Input: part model. Units: mm. Frame: model coordinates. Coordinates: 2 decimals unless noted, no trailing zeros. Loops run counter-clockwise (first coordinate to the right, second up) from the corner with the lowest first, then second, coordinate; pieces in that order, holes last. Notation, with made-up numbers: (5.25, 38) - (52.25, 38) arc R26 cw to (52.25, 58) - close; hole circle Ø6 at (33, 56.25). An arc over 180 degrees is marked (long way). Use a Markdown table: item, result. Add a question column.
1. Draft query along Y for faces 1 (the face through (-1, 1, 0)), 2 (the face through (0.221, -18.314, 0.606)), 3 (the face through (-8.67, -39.05, 1.48)). Return one class per face: released by +Y, released by -Y, zero draft, split by the parting line, or undercut.
2. Section query C-C on y = -20. Return the cut outline in (x, z), then the cut area to 3 significant figures.
3. Contact query for flat-ended pins moving along their axis: P1, Ø4.5, axis at x = 20, y = 0, coming from the +Z side; P2, Ø4, axis at x = 0, y = -20, coming from the +Z side; P3, Ø2.5, axis at x = 0, y = 20, coming from the +Z side; P4, Ø1, axis at y = -26.5, z = 1, coming from the +X side. Output: stop coordinate, or through.
4. Section query A-A on z = 1.8. Return the cut outline in (x, y).
5. Section query B-B on x = 0. Return the cut outline in (y, z).
6. Ray query, L1, parallel to Y at x = 0, z = 0.7; L2, parallel to Y at x = -20, z = 0.75. Return the intervals inside material, ascending. Write a range as [from, to].
```python
from build123d import *

# Parameters (mm, degrees)
SKETCH_1_R                   = 40
EXTRUDE_1_DEPTH              = 3
HOLE_WIZARD_M3_1_D           = 3.4
HOLE_WIZARD_M3_1_DEPTH       = 10.12
HOLE_WIZARD_M3_1_CSINK_D     = 6.94
HOLE_WIZARD_M3_1_CSINK_ANGLE = 90
HOLE_WIZARD_M3_1_TIP         = 1.021463052


with BuildPart() as part:
    # 草图1 → 凸台-拉伸1 (new body)
    with BuildSketch(Plane.XY):
        Circle(SKETCH_1_R)
    extrude(amount=EXTRUDE_1_DEPTH)

    # M3 六角凹锥坑头螺钉的锥形沉头孔1
    with Locations(Plane(origin=(0, 20, 3), x_dir=(1, 0, 0), z_dir=(0, 0, 1))):
        with Locations((0, 0), (20, -20), (0, -40), (-20, -20)):
            CounterSinkHole(HOLE_WIZARD_M3_1_D / 2, HOLE_WIZARD_M3_1_CSINK_D / 2, depth=HOLE_WIZARD_M3_1_DEPTH, counter_sink_angle=HOLE_WIZARD_M3_1_CSINK_ANGLE)
            with Locations((0, 0, -(HOLE_WIZARD_M3_1_DEPTH + HOLE_WIZARD_M3_1_TIP / 2))):  # 118° drill point
                Cone(0, HOLE_WIZARD_M3_1_D / 2, HOLE_WIZARD_M3_1_TIP, mode=Mode.SUBTRACT)


solid = part.part
```
Resolved:
| question | item | result |
|---|---|---|
| 1 | face 1 | zero draft |
| 1 | face 2 | undercut |
| 1 | face 3 | split by the parting line |
| 2 | outline | (-34.64, 0) - (-1.7, 0) - (-1.7, 1.23) - (-3.47, 3) - (-34.64, 3) - close; (1.7, 0) - (34.64, 0) - (34.64, 3) - (3.47, 3) - (1.7, 1.23) - close |
| 2 | area | 195 mm² |
| 3 | P1 | z = 1.78 |
| 3 | P2 | z = 1.53 |
| 3 | P3 | through |
| 3 | P4 | x = 30.4 |
| 4 | outline | circle Ø80 at (0, 0); hole circle Ø4.54 at (-20, 0); hole circle Ø4.54 at (0, -20); hole circle Ø4.54 at (0, 20); hole circle Ø4.54 at (20, 0) |
| 5 | outline | (-40, 0) - (-21.7, 0) - (-21.7, 1.23) - (-23.47, 3) - (-40, 3) - close; (-18.3, 0) - (18.3, 0) - (18.3, 1.23) - (16.53, 3) - (-16.53, 3) - (-18.3, 1.23) - close; (21.7, 0) - (40, 0) - (40, 3) - (23.47, 3) - (21.7, 1.23) - close |
| 6 | L1 | [-40, -21.7], [-18.3, 18.3], [21.7, 40] |
| 6 | L2 | [-34.64, -1.7], [1.7, 34.64] |
